Could you check a few things on this model? Use its own coordinates, in mm. Give positions to 0.01 mm unless a question says otherwise; leave off trailing zeros. Order: outer loops, then holes, each group sorted by start corner. A loop starts at its lowest first (then second) coordinate and runs counter-clockwise, first axis right, second up. Notation, with made-up numbers: M -31,-9 L 7,-9 A19 cw 7,1 Z; hole C 61.5,55 d7. An arc over 180 degrees is marked long. Answer in a Markdown table with one row per item. Add a question column.
```python
from build123d import *

# Parameters (mm, degrees)
EXTRUDE_1_DEPTH     = 0.7
SKETCH_2_R          = 4.05
EXTRUDE_2_DEPTH     = 3
SKETCH_3_W          = 5.2
SKETCH_3_H          = 4.2
CUT_EXTRUDE_1_DEPTH = 0.01
SKETCH_4_R          = 0.25
EXTRUDE_3_DEPTH     = 4


with BuildPart() as part:
    # Эскиз1 → Бобышка-Вытянуть1 (new body)
    with BuildSketch(Plane.XY):
        with BuildLine():
            Line((5.2, 0.4), (4.582575695, 0.4))
            ThreePointArc((4.582575695, 0.4), (-4.6, 0), (4.582575695, -0.4))
            Line((4.582575695, -0.4), (5.2, -0.4))
            ThreePointArc((5.2, -0.4), (5.6, 0), (5.2, 0.4))
        make_face()
    extrude(amount=EXTRUDE_1_DEPTH)

    # Эскиз2 → Бобышка-Вытянуть2 (add)
    with BuildSketch(Plane.XY.offset(0.7)):
        Circle(SKETCH_2_R)
    extrude(amount=EXTRUDE_2_DEPTH)

    # Эскиз3 → Вырез-Вытянуть1 (cut)
    with BuildSketch(Plane.XY.offset(3.7)):
        Rectangle(SKETCH_3_W, SKETCH_3_H)
    extrude(amount=-CUT_EXTRUDE_1_DEPTH, mode=Mode.SUBTRACT)

    # Эскиз4 → Бобышка-Вытянуть3 (add)
    with BuildSketch(Plane.XY):
        with Locations((1.796, 1.796)):
            Circle(SKETCH_4_R)
        with Locations((-1.796, 1.796)):
            Circle(SKETCH_4_R)
        with Locations((-1.796, -1.796)):
            Circle(SKETCH_4_R)
    extrude(amount=-EXTRUDE_3_DEPTH)


solid = part.part
```
1. Suppose I cut it at D-D on z = 2.25. List the corners of the cut face in (x, y) for me, plus the area to 3 significant figures.
2. Suppose I cut it at C-C on z = -1. List the corners of the cut face in (x, y) for me, plus the area to 3 significant figures.
3. Will these pins go through, and if not, where does the flat tip stop? P1, Ø0.7, axis at x = 5, z = 0.5, coming from the +Y side; P2, Ø2, axis at x = 1.5, y = -1, coming from the -Z side; P3, Ø1.3, axis at x = 1, y = 0.5, coming from the +Z side.
4. If I drill on line 1 along Z through (x, y) = (3.5, -1.25); line 2 along Y through (x, z) = (1.75, 2.25); line 3 along Y through (x, z) = (0.25, 2), over which ranges is the centre line in solid material (lowest first)? Write a range as [from, to].
5. Thinking about a two-plate mould opening in Y: for faces 1 (the cylindrical face through (-4.596, 0.197, 0.345)), 2 (the flat face through (3, 0, 3.7)), 3 (the flat face through (0, 0, 3.69)), which applies, pulls with the +Y half, pulls with the -Y half, needs draft (parallel to the pull), parting line crosses it, or undercut?
Findings below:
| question | item | result |
|---|---|---|
| 1 | outline | C 0,0 d8.1 |
| 1 | area | 51.5 mm2 |
| 2 | outline | C -1.8,-1.8 d0.5; C -1.8,1.8 d0.5; C 1.8,1.8 d0.5 |
| 2 | area | 0.589 mm2 |
| 3 | P1 | y = 0.4 |
| 3 | P2 | z = 0 |
| 3 | P3 | z = 3.69 |
| 4 | line 1 | [0, 3.7] |
| 4 | line 2 | [-3.65, 3.65] |
| 4 | line 3 | [-4.04, 4.04] |
| 5 | face 1 | parting line crosses it |
| 5 | face 2 | needs draft |
| 5 | face 3 | undercut |
